from build123d import *

# Parameters (mm, degrees)
SKETCH1_R           = 90
BOSS_EXTRUDE1_DEPTH = 30
SKETCH2_R           = 50
CUT_EXTRUDE1_DEPTH  = 70
SKETCH3_R           = 10
CUT_EXTRUDE2_DEPTH  = 70


with BuildPart() as part:
    # Sketch1 → Boss-Extrude1 (new body)
    with BuildSketch(Plane.XY):
        Circle(SKETCH1_R)
    extrude(amount=BOSS_EXTRUDE1_DEPTH)

    # Sketch2 → Cut-Extrude1 (cut)
    with BuildSketch(Plane.XY):
        Circle(SKETCH2_R)
    extrude(amount=CUT_EXTRUDE1_DEPTH, mode=Mode.SUBTRACT)

    # Sketch3 → Cut-Extrude2 (cut)
    with BuildSketch(Plane.XY.offset(30)):
        with Locations((70, 0)):
            Circle(SKETCH3_R)
    extrude(amount=-CUT_EXTRUDE2_DEPTH, mode=Mode.SUBTRACT)


solid = part.part
Verification items for the finished model (mm, model axes). Coordinates: 2 decimals unless noted, no trailing zeros. Order: outer loops, then holes, each group sorted by start corner. A loop starts at its lowest first (then second) coordinate and runs counter-clockwise, first axis right, second up. Notation, with made-up numbers: M -25.75,10 L 15.25,10 A36 ccw 15.25,47 Z; hole C 85.5,-32.5 d8. An arc over 180 degrees is marked long. One line per item, written item: value. Start each with the question number.
Item 1: Mould release check, pull along Y, two halves, no side actions. Record for faces 1 (the cylindrical face through (41.53, -79.845, 14.79)), 2 (the flat face through (39, -39, 30)), 3 (the cylindrical face through (60, 0, 15)): released by +Y, released by -Y, zero draft, split by the parting line, or undercut.
Item 2: Sectioned sample at B-B (x = 70). Enter the section's corners in (y, z).
Item 3: Scan lines: probe 1 along Y at (x, z) = (0, 12.5); probe 2 along X at (y, z) = (-34, 15.25); probe 3 along X at (y, z) = (7, 11). Record each from-to range of solid material in increasing order.
Item 4: Sectioned sample at C-C (z = 21.75). Enter the section's corners in (x, y), then the cut area to 3 significant figures.
Item 5: Sectioned sample at A-A (y = 0). Enter the section's corners in (x, z), then the cut area to 3 significant figures.
Item 6: Gauge pin test, flat ends, axial feed: pin 1 (3 mm diameter, centred on x = 15, z = 6.5, fed in from +Y); pin 2 (1.5 mm diameter, centred on y = 1, z = 13, fed in from -X); pin 3 (12 mm diameter, centred on y = 29, z = 16, fed in from -X). Record the tip position at first contact, or that the pin passes through.
Item 7: Sectioned sample at D-D (x = 0). Enter the section's corners in (y, z), then the cut area to 3 significant figures.
Conclusion:
1. face 1: split by the parting line
1. face 2: zero draft
1. face 3: undercut
2. outline: M -56.57,0 L -10,0 L -10,30 L -56.57,30 Z; M 10,0 L 56.57,0 L 56.57,30 L 10,30 Z
3. probe 1: y = -90 to -50, 50 to 90
3. probe 2: x = -83.33 to -36.66, 36.66 to 83.33
3. probe 3: x = -89.73 to -49.51, 49.51 to 62.86, 77.14 to 89.73
4. outline: C 0,0 d180; hole C 0,0 d100; hole C 70,0 d20
4. area: 17,300 mm^2
5. outline: M -90,0 L -50,0 L -50,30 L -90,30 Z; M 50,0 L 60,0 L 60,30 L 50,30 Z; M 80,0 L 90,0 L 90,30 L 80,30 Z
5. area: 1,800 mm^2
6. pin 1: stops at y = 88.98
6. pin 2: stops at x = -90
6. pin 3: stops at x = -87.01
7. outline: M -90,0 L -50,0 L -50,30 L -90,30 Z; M 50,0 L 90,0 L 90,30 L 50,30 Z
7. area: 2,400 mm^2
